Autodesk Inventor part; units mm, degrees
ref_plane "YZ Plane" through (0, 0, 0) normal (1, 0, 0) x (0, 1, 0)
ref_plane "XZ Plane" through (0, 0, 0) normal (0, 1, 0) x (-1, 0, 0)
ref_plane "XY Plane" through (0, 0, 0) normal (0, 0, 1) x (1, 0, 0)
sketch "Skizze1" plane through (0, 0, 0) normal (0, 0, 1) x (1, 0, 0)
  circle A0 centre (0, 0) radius 2.25
  line L0 (0, 4.25) -> (-6, 4.25)
  line L1 (-6, 4.25) -> (-6, -13.5)
  line L2 (-6, -13.5) -> (-4, -13.5)
  line L3 (-4, -13.5) -> (-4, -19.5)
  line L4 (-4, -19.5) -> (0, -19.5)
  line L5 (0, -19.5) -> (0, -4.25)
  arc A1 (0, -4.25) -> (0, 4.25) centre (0, 0) ccw
  line L6 (0, 9) -> (0, -24.25)
  line L7 (-8.05, 0) -> (6.3, 0)
  dimension "d0" = 4.5
  dimension "d1" = 4
  dimension "d2" = 2
  dimension "d3" = 2
  dimension "d4" = 13.5
  dimension "d5" = 6
extrude "Extrusion1" add sketch "Skizze1" along normal blind 20 contours L7 A1 L6 A0 | A0 L6 A1 L7 | A0 L7 L1 L0 L6 | L6 L5 L4 L3 L2 L1 L7 A0
sketch "Skizze2" plane through (-6, -13.5, 0) normal (-1, 0, 0) x (0, 0, 1)
  line L0 (20, 0) -> (20, 17.75)
  line L1 (0, 17.75) -> (0, 0)
  line L2 (0, 15.75) -> (20, 15.75)
  line L3 (0, 11.25) -> (20, 11.25)
  point P0 (0, 13.5)
  point P1 (4, 13.5)
  point P2 (16, 13.5)
  dimension "d8" = 4
  dimension "d9" = 4
hole "Bohrung1" at (-6, 0, 4) at (-6, 0, 16) direction (1, 0, 0) diameter 1.567 end up to surface
sketch "Skizze3" plane through (-4, -19.5, 0) normal (-1, 0, 0) x (0, 0, 1)
  line L0 (20, 0) -> (20, 6)
  line L1 (0, 6) -> (0, 0)
  point P0 (0, 19.5)
  point P1 (4, 3)
  point P2 (16, 3)
  dimension "d17" = 4
  dimension "d18" = 4
hole "Bohrung2" at (-4, -16.5, 4) at (-4, -16.5, 16) direction (1, 0, 0) diameter 1.567 end up to surface
fillet "Rundung1" radius 2 1 edges at (-6, 4.25, 10)
fillet "Rundung2" radius 3 1 edges at (0, -4.25, 10)
properties part number "Türarm"
Geometry check sheet. Reference: the model listing, model coordinates, mm. A direction names the side the tool comes from. Coordinates: 2 decimals unless noted, no trailing zeros. Order: outer loops, then holes, each group sorted by start corner. A loop starts at its lowest first (then second) coordinate and runs counter-clockwise, first axis right, second up. Notation, with made-up numbers: (-10.5, 11) - (17.5, 11) arc R33 cw to (17.5, 44) - close; hole circle Ø4 at (82, 82). An arc over 180 degrees is marked (long way). One line per item, written item: value.
(1) Access from +Z, -Z, +X, -X, +Y, -Y to the whole of each face (thin tool, end or side, straight path). Record for faces 5 (the face through (0, -13, 10)), 6 (the face through (-4.027, 0.3, 16.724)), 7 (the face through (-5.4, 3.68, 10.14)), 8 (the face through (-5, -13.5, 10)).
Data:
face 5: +Z, -Z, +X, -Y
face 6: -X
face 7: +Z, -Z, -X, +Y
face 8: +Z, -Z, -X, -Y
(2) Release check for a two-part mould opening along Z. For faces 1 (the face through (-4.027, 0.3, 4.724)), 2 (the face through (-1.972, -15.805, 4.362)), 3 (the face through (2.146, -0.676, 9.86)), 4 (the face through (-2, -5, 20)) record: +Z half, -Z half, draft (parallel to the pull), parting line (faces both ways), or undercut.
Data:
face 1: undercut
face 2: undercut
face 3: draft
face 4: +Z half
(3) Sectioned sample at D-D (x = -2.75). Enter the section's corners in (y, z), and give its area (3 significant figures).
Data:
outline: (-19.5, 0) - (4.25, 0) - (4.25, 20) - (-19.5, 20) - close; hole circle Ø1.57 at (-16.5, 4); hole circle Ø1.57 at (-16.5, 16); hole circle Ø1.57 at (0, 4); hole circle Ø1.57 at (0, 16)
area: 467 mm^2
(4) Sectioned sample at A-A (x = -1). Enter the section's corners in (y, z), and give its area (3 significant figures).
Data:
outline: (-19.5, 0) - (-2.02, 0) - (-2.02, 20) - (-19.5, 20) - close; (2.02, 0) - (4.25, 0) - (4.25, 20) - (2.02, 20) - close; hole circle Ø1.57 at (-16.5, 4); hole circle Ø1.57 at (-16.5, 16)
area: 391 mm^2
(5) Thickness scan on probe 1 along Z at (x, y) = (-1.1, -16.5); probe 2 along X at (y, z) = (0, 7.5); probe 3 along X at (y, z) = (-15.5, 12.75). Record the ranges inside material, lowest first. Write a range as from..to.
Data:
probe 1: z = 0..3.22, 4.78..15.22, 16.78..20
probe 2: x = -6..-2.25, 2.25..4.25
probe 3: x = -4..0
(6) Sectioned sample at C-C (z = 4). Enter the section's corners in (x, y).
Data:
outline: (-6, -13.5) - (-4, -13.5) - (-4, -15.72) - (0, -15.72) - (0, -6.6) arc R3 cw to (1.76, -3.87) arc R4.25 ccw to (0, 4.25) - (-4, 4.25) arc R2 ccw to (-6, 2.25) - (-6, 0.78) - (-2.11, 0.78) arc R2.25 cw (long way) to (-2.11, -0.78) - (-6, -0.78) - close; (-4, -19.5) - (0, -19.5) - (0, -17.28) - (-4, -17.28) - close
(7) Sectioned sample at B-B (y = -16.5). Enter the section's corners in (x, z).
Data:
outline: (-4, 0) - (0, 0) - (0, 3.22) - (-4, 3.22) - close; (-4, 4.78) - (0, 4.78) - (0, 15.22) - (-4, 15.22) - close; (-4, 16.78) - (0, 16.78) - (0, 20) - (-4, 20) - close
(8) Depth check by flat-ended pin: pin 1 Ø2 at (y, z) = (-16.5, 4) entering from -X; pin 2 Ø0.6 at (x, z) = (-5, 8) entering from -Y; pin 3 Ø1.5 at (x, z) = (1.5, 13.5) entering from +Y; pin 4 Ø1.4 at (y, z) = (-16.5, 16) entering from +X. Enter the tip coordinate at first touch or a pass-through.
Data:
pin 1: stops at x = -4
pin 2: stops at y = -13.5
pin 3: stops at y = 4.18
pin 4: passes through
